from build123d import *

# Parameters (mm, degrees)
SKETCH1_W                      = 160
SKETCH1_H                      = 100
BOSS_EXTRUDE1_DEPTH            = 40
SKETCH2_W                      = 65
SKETCH2_H                      = 90
CUT_EXTRUDE1_DEPTH             = 25
FILLET1_R                      = 8
SKETCH3_W                      = 60
SKETCH3_H                      = 38
SKETCH3_W_2                    = 38
SKETCH3_H_2                    = 25
CUT_EXTRUDE2_DEPTH             = 20
FILLET2_R                      = 6
FILLET3_R                      = 8
FILLET4_R                      = 10
CBORE_FOR_M6_SHCS1_D           = 6.6
CBORE_FOR_M6_SHCS1_CBORE_D     = 11
CBORE_FOR_M6_SHCS1_CBORE_DEPTH = 6


with BuildPart() as part:
    # Sketch1 → Boss-Extrude1 (new body)
    with BuildSketch(Plane.XY):
        Rectangle(SKETCH1_W, SKETCH1_H)
    extrude(amount=-BOSS_EXTRUDE1_DEPTH)

    # Sketch2 → Cut-Extrude1 (cut)
    with BuildSketch(Plane.XY):
        with Locations((-40, 0)):
            Rectangle(SKETCH2_W, SKETCH2_H)
    extrude(amount=-CUT_EXTRUDE1_DEPTH, mode=Mode.SUBTRACT)

    # Fillet1
    fillet1_edges = [part.edges().sort_by_distance(p)[0] for p in [
        (-7.5, 45, -12.5),
        (-7.5, -45, -12.5),
        (-72.5, -45, -12.5),
        (-72.5, 45, -12.5),
    ]]
    fillet(fillet1_edges, radius=FILLET1_R)

    # Sketch3 → Cut-Extrude2 (cut)
    with BuildSketch(Plane.XY):
        with Locations((40, -25)):
            Rectangle(SKETCH3_W, SKETCH3_H)
        with Locations((40, 25)):
            Rectangle(SKETCH3_W_2, SKETCH3_H_2)
    extrude(amount=-CUT_EXTRUDE2_DEPTH, mode=Mode.SUBTRACT)

    # Fillet2
    fillet2_edges = [part.edges().sort_by_distance(p)[0] for p in [
        (59, 37.5, -10),
        (59, 12.5, -10),
        (21, 12.5, -10),
        (21, 37.5, -10),
    ]]
    fillet(fillet2_edges, radius=FILLET2_R)

    # Fillet3
    fillet3_edges = [part.edges().sort_by_distance(p)[0] for p in [
        (70, -6, -10),
        (70, -44, -10),
        (10, -44, -10),
        (10, -6, -10),
    ]]
    fillet(fillet3_edges, radius=FILLET3_R)

    # Fillet4
    fillet4_edges = [part.edges().sort_by_distance(p)[0] for p in [
        (80, -50, -20),
        (-80, -50, -20),
        (-80, 50, -20),
        (80, 50, -20),
    ]]
    fillet(fillet4_edges, radius=FILLET4_R)

    # CBORE for M6 SHCS1 (through all)
    with Locations(Plane.XY):
        with Locations((2.910260727, 0)):
            CounterBoreHole(CBORE_FOR_M6_SHCS1_D / 2, CBORE_FOR_M6_SHCS1_CBORE_D / 2, CBORE_FOR_M6_SHCS1_CBORE_DEPTH)


solid = part.part
Design review of the part built by this model. Coordinates are the model's own, in mm. A direction names the side the tool comes from. Coordinates: 2 decimals unless noted, no trailing zeros. Loops run counter-clockwise (first coordinate to the right, second up) from the corner with the lowest first, then second, coordinate; pieces in that order, holes last. Notation, with made-up numbers: M -34.75,64.25 L -16.75,64.25 A15 ccw -16.75,71.25 Z; hole C 26,82 d1. An arc over 180 degrees is marked long. Use one line per item in the form item = value.
(1) Clearance check with flat-ended pins moving along their axes: P1, Ø8, axis at x = -37.5, y = -18, coming from the +Z side; P2, Ø10.5, axis at x = 2.91, y = 0, coming from the -Z side; P3, Ø5.5, axis at x = 3.5, y = 2.5, coming from the +Z side. State where each tip first meets the part, or that it passes through.
Return value:
P1 = -25
P2 = -40
P3 = -6
(2) Draft analysis for pull direction Y (two halves, no side actions). For faces 1 (the face through (-77.15, 46.99, -20.28)), 2 (the face through (40, -6, -10)), 3 (the face through (80, -1, -20)), 4 (the face through (12.406, -8.281, -10.14)), state which applies: pulls with the +Y half, pulls with the -Y half, needs draft (parallel to the pull), parting line crosses it, or undercut.
Return value:
face_1 = pulls with the +Y half
face_2 = undercut
face_3 = needs draft
face_4 = undercut
(3) For line 1 along X through (y, z) = (-21.5, -15.5); line 2 along Y through (x, z) = (28.5, -15.5); line 3 along X through (y, z) = (6, -12), list the stretches that pass through material, from the lowest coordinate up. Write a range as from..to.
Return value:
line_1 = -80..-72.5, -7.5..10, 70..80
line_2 = -50..-44, -6..12.5, 37.5..50
line_3 = -80..-72.5, -7.5..80
(4) Consider section D-D (x = 3.5). Write out the cut boundary in (y, z).
Return value:
outline = M -50,-40 L -3.25,-40 L -3.25,-6 L -5.47,-6 L -5.47,0 L -50,0 Z; M 3.25,-40 L 50,-40 L 50,0 L 5.47,0 L 5.47,-6 L 3.25,-6 Z
(5) Consider section A-A (z = -12.5). Give the number of separate pieces and of enclosed holes in the cut face, and give its area (3 significant figures).
Return value:
separate_pieces = 1
enclosed_holes = 4
area = 6,940 mm2
(6) Consider section B-B (y = 0). Write out the cut boundary in (x, z), and give its area (3 significant figures).
Return value:
outline = M -80,-40 L -0.39,-40 L -0.39,-6 L -2.59,-6 L -2.59,0 L -7.5,0 L -7.5,-25 L -72.5,-25 L -72.5,0 L -80,0 Z; M 6.21,-40 L 80,-40 L 80,0 L 8.41,0 L 8.41,-6 L 6.21,-6 Z
area = 4,480 mm2
(7) For faces 5 (the face through (59, 25, -10)), 6 (the face through (-0.237, 0.991, -23.238)), list the 3-axis set-ups (+Z, -Z, +X, -X, +Y, -Y) from which the entire face can be reached by the end or side of a thin tool; tool diameter is ignored.
Return value:
face_5 = +Z
face_6 = +Z, -Z
(8) Consider section C-C (x = -21). Write out the cut boundary in (y, z), and give its area (3 significant figures).
Return value:
outline = M -50,-40 L 50,-40 L 50,0 L 45,0 L 45,-25 L -45,-25 L -45,0 L -50,0 Z
area = 1,750 mm2
